Check sheet for the drawn part. Datum: minimum x, y, z corner. Units: mm. A direction names the side the tool comes from. Round coordinates to 2 decimals unless told otherwise and drop trailing zeros. Order: outer loops, then holes, each group sorted by start corner. A loop starts at its lowest first (then second) coordinate and runs counter-clockwise, first axis right, second up.
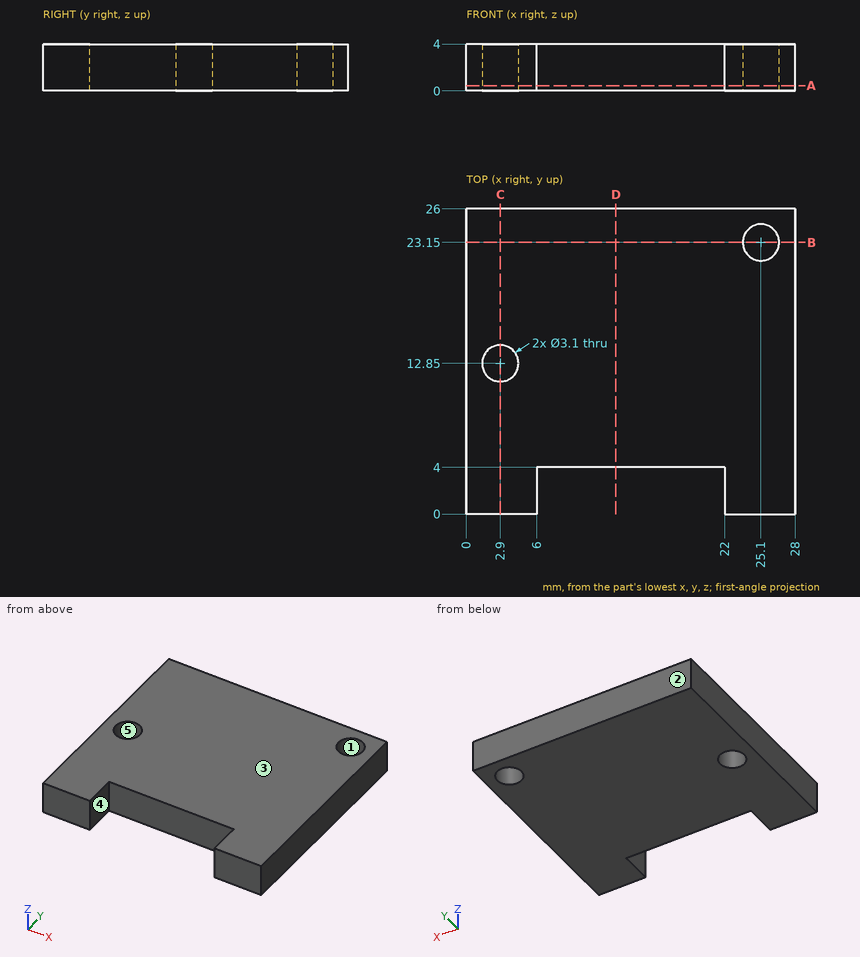
(1) Sectioned sample at C-C, the plane x = 2.9. Record the cut outline in (y, z), and give its area (3 significant figures).
Returned:
outline: (0, 0) - (11.3, 0) - (11.3, 4) - (0, 4) - close; (14.4, 0) - (26, 0) - (26, 4) - (14.4, 4) - close
area: 91.6 mm2
(2) Draft check along Y on the marked faces 1, 2 and 3. Enter one of: released by +Y, released by -Y, zero draft, split by the parting line, or undercut.
Returned:
face 1: undercut
face 2: released by +Y
face 3: zero draft
(3) Material ranges on line 1 (Y direction, x = 2.9, z = 1.75); line 2 (Y direction, x = 25.1, z = 2.5); line 3 (X direction, y = 1, z = 3), recorded low to high.
Returned:
line 1: y = 0 to 11.3, 14.4 to 26
line 2: y = 0 to 21.6, 24.7 to 26
line 3: x = 0 to 6, 22 to 28
(4) Depth check by flat-ended pin: P1, Ø2, axis at x = 13, z = 2.5, coming from the -Y side. Enter the tip coordinate at first touch or a pass-through.
Returned:
P1: stops at y = 4
(5) Set-up check for the marked faces 4 and 5: record each of +Z, -Z, +X, -X, +Y, -Y from which the full face is reachable in a straight line by a thin tool's end or side.
Returned:
face 4: +Z, -Z, -Y
face 5: +Z, -Z
(6) Sectioned sample at A-A, the plane z = 0.45. Record the cut outline in (x, y).
Returned:
outline: (0, 0) - (6, 0) - (6, 4) - (22, 4) - (22, 0) - (28, 0) - (28, 26) - (0, 26) - close; hole circle Ø3.1 at (2.9, 12.85); hole circle Ø3.1 at (25.1, 23.15)
(7) Sectioned sample at B-B, the plane y = 23.15. Record the cut outline in (x, z).
Returned:
outline: (0, 0) - (23.55, 0) - (23.55, 4) - (0, 4) - close; (26.65, 0) - (28, 0) - (28, 4) - (26.65, 4) - close
(8) Sectioned sample at D-D, the plane x = 12.75. Record the cut outline in (y, z).
Returned:
outline: (4, 0) - (26, 0) - (26, 4) - (4, 4) - close
